Autodesk Inventor part; units mm, degrees
ref_plane "YZ Plane" through (0, 0, 0) normal (1, 0, 0) x (0, 1, 0)
ref_plane "XZ Plane" through (0, 0, 0) normal (0, 1, 0) x (-1, 0, 0)
ref_plane "XY Plane" through (0, 0, 0) normal (0, 0, 1) x (1, 0, 0)
sketch "Sketch1" plane through (0, 0, 0) normal (0, 0, 1) x (1, 0, 0)
  line L0 (0, 0) -> (-6.35, 6.35)
  line L1 (-6.35, 6.35) -> (-103.1386, 3.175)
  line L2 (-103.1386, -3.175) -> (-6.35, -6.35)
  line L3 (-6.35, -6.35) -> (0, 0)
  arc A0 (-103.1386, 3.175) -> (-103.1386, -3.175) centre (0, 0) ccw
  line L4 (0, 0) -> (0.1245, 0) construction
  dimension "d1" = 6.35
  dimension "d3" = 6.35
  dimension "d10" = 135
  dimension "d11" = 103.1875
extrude "Extrusion1" add sketch "Sketch1" along normal blind 6.35
fillet "Fillet2" radius 3.81 2 edges at (-54.7443, -4.7625, 6.35) (-54.7443, 4.7625, 6.35)
hole "Hole1" at (0, 0, 6.35) direction (0, 0, -1) diameter 3.175 depth 25.4 tip angle 118
properties part number "Thrust_Support"
The model under review builds one solid part; all positions refer to its coordinate system, in mm. Coordinates: 2 decimals unless noted, no trailing zeros.
1) Clearance check with a flat-ended pin moving along its axis: pin 1 Ø5 at (x, y) = (-73, -3) entering from +Z. State where the tip first meets the part, or that it passes through.
2) To check wall thickness, follow probe 1 along Z at (x, y) = (-92.5, -0.25); probe 2 along X at (y, z) = (0, 2.5); probe 3 along Y at (x, z) = (-64, 3). State the ranges of each line that lie inside material, in increasing order.
3) The part is to be moulded in two halves that separate along Y. For faces 1 (the face through (-1.587, -0.017, 3.131)), 2 (the face through (-42, 0, 0)), 3 (the face through (-52.3, 3.76, 5.2)), 4 (the face through (-53.706, -3.71, 5.204)), say which applies: pulls with the +Y half, pulls with the -Y half, needs draft (parallel to the pull), parting line crosses it, or undercut.
Answer list:
1. pin 1: stops at z = 6.35
2. probe 1: z = 0 to 6.31
2. probe 2: x = -103.19 to -1.59
2. probe 3: y = -4.43 to 4.43
3. face 1: undercut
3. face 2: needs draft
3. face 3: pulls with the +Y half
3. face 4: pulls with the -Y half
